from build123d import *

# Parameters (mm, degrees)
SKETCH1_R           = 42.5
SKETCH1_R_2         = 35.5
BOSS_EXTRUDE3_DEPTH = 20
BOSS_EXTRUDE4_DEPTH = 20
BOSS_EXTRUDE6_DEPTH = 20


with BuildPart() as part:
    # Sketch1 → Boss-Extrude3 (new body)
    with BuildSketch(Plane(origin=(0, 0, 0), x_dir=(1, 0, 0), z_dir=(0, 1, 0))):
        Circle(SKETCH1_R)
        Circle(SKETCH1_R_2, mode=Mode.SUBTRACT)
    extrude(amount=BOSS_EXTRUDE3_DEPTH)

    # Sketch5 → Boss-Extrude4 (add)
    with BuildSketch(Plane(origin=(0, 0, 0), x_dir=(1, 0, 0), z_dir=(0, 1, 0))):
        with BuildLine():
            Line((-30, -94.285), (30, -94.285))
            Line((30, -94.285), (30, -30.103986447))
            ThreePointArc((30, -30.103986447), (0, -42.5), (-30, -30.103986447))
            Line((-30, -30.103986447), (-30, -94.285))
        make_face()
    extrude(amount=BOSS_EXTRUDE4_DEPTH)

    # Sketch6 → Boss-Extrude6 (add)
    with BuildSketch(Plane.XY.offset(94.285)):
        with BuildLine():
            Line((70, -20), (-70, -20))
            ThreePointArc((-70, -20), (-100, 10), (-70, 40))
            Line((-70, 40), (70, 40))
            ThreePointArc((70, 40), (100, 10), (70, -20))
        make_face()
        with BuildLine():
            Line((-45, 0), (-75, 0))
            ThreePointArc((-75, 0), (-85, 10), (-75, 20))
            Line((-75, 20), (-45, 20))
            ThreePointArc((-45, 20), (-35, 10), (-45, 0))
        make_face(mode=Mode.SUBTRACT)
        with BuildLine():
            Line((45, 0), (75, 0))
            ThreePointArc((75, 0), (85, 10), (75, 20))
            Line((75, 20), (45, 20))
            ThreePointArc((45, 20), (35, 10), (45, 0))
        make_face(mode=Mode.SUBTRACT)
    extrude(amount=BOSS_EXTRUDE6_DEPTH)


solid = part.part
Can you work these out from the model? Positions are in its coordinate system, mm. A direction names the side the tool comes from. Coordinates: 2 decimals unless noted, no trailing zeros. Write each loop counter-clockwise with the first axis right and the second up, starting at its lowest first coordinate (ties: lowest second). Pieces come first, ordered by that corner, then holes. Notation, with made-up numbers: (-26, -18.75) -> (-14, -18.75) arc R23 cw to (-14, 15.25) -> close; hole circle Ø6 at (71.5, 18). An arc over 180 degrees is marked (long way). Write each question's results on one line, items separated by ' | '. Start each with the question number.
Item 1: If we section it at A-A, the plane y = 10: Write out the boundary of the cut face in (x, z) (3 decimals).
Item 2: Thinking about a two-plate mould opening in X: for faces 5 (the flat face through (-30, 10, 62)), 6 (the cylindrical face through (85, 10, 104)), 7 (the flat face through (-60, 0, 104)), 8 (the flat face through (-1, 0, 40)), which applies, released by +X, released by -X, zero draft, split by the parting line, or undercut?
Item 3: Please list where these lines run through material, in increasing order: probe 1 along X at (y, z) = (8.75, 0); probe 2 along Z at (x, y) = (0, 14) (3 decimals); probe 3 along Z at (x, y) = (-85, -2.5) (3 decimals).
Item 4: If we section it at D-D, the plane z = 98: Write out the boundary of the cut face in (x, y).
Item 5: On a 3-axis mill with a long thin cutter (end or side, diameter ignored), from which of +Z, -Z, +X, -X, +Y, -Y can I reach the whole of each face in a straight line? I mean faces 1 (the flat face through (-1, 20, 40)), 2 (the flat face through (30, 10, 63)), 3 (the cylindrical face through (35, 10, 104)), 4 (the flat face through (-60, 20, 104)). Say none if no direction works.
Item 6: If we section it at C-C, the plane x = 48: Write out the boundary of the cut face in (y, z) (3 decimals).
Item 7: I'm going to push flat-ended pins straight in: P1, Ø10, axis at y = 22.5, z = -5.5, coming from the +X side; P2, Ø6, axis at x = -46, y = 15.5, coming from the +Z side; P3, Ø6, axis at y = 14, z = 64.5, coming from the +X side; P4, Ø16, axis at y = 11, z = 77.5, coming from the -X side. Where does each tip first touch, or does it pass through?
Item 8: If we section it at B-B, the plane z = 0: Write out the boundary of the cut face in (x, y), and give its area (3 significant figures).
Answer block:
1) outline: (-100, 94.285) -> (-85, 94.285) -> (-85, 114.285) -> (-100, 114.285) -> close; (-35, 94.285) -> (-30, 94.285) -> (-30, 30.104) arc R42.5 ccw (long way) to (30, 30.104) -> (30, 94.285) -> (35, 94.285) -> (35, 114.285) -> (-35, 114.285) -> close; (85, 94.285) -> (100, 94.285) -> (100, 114.285) -> (85, 114.285) -> close; hole circle Ø71 at (0, 0)
2) face 5: released by -X | face 6: undercut | face 7: undercut | face 8: zero draft
3) probe 1: -42.5 to -35.5, 35.5 to 42.5 | probe 2: -42.5 to -35.5, 35.5 to 114.285 | probe 3: 94.285 to 114.285
4) outline: (-70, -20) -> (70, -20) arc R30 ccw to (70, 40) -> (-70, 40) arc R30 ccw to start; hole (-75, 0) -> (-45, 0) arc R10 ccw to (-45, 20) -> (-75, 20) arc R10 ccw to start; hole (45, 0) -> (75, 0) arc R10 ccw to (75, 20) -> (45, 20) arc R10 ccw to start
5) face 1: -Z, +X, -X, +Y | face 2: +X, +Y, -Y | face 3: +Z | face 4: +Z, -Z
6) outline: (-20, 94.285) -> (0, 94.285) -> (0, 114.285) -> (-20, 114.285) -> close; (20, 94.285) -> (40, 94.285) -> (40, 114.285) -> (20, 114.285) -> close
7) P1: x = 42.48 | P2: through | P3: x = 30 | P4: x = -30
8) outline: (-42.5, 0) -> (-35.5, 0) -> (-35.5, 20) -> (-42.5, 20) -> close; (35.5, 0) -> (42.5, 0) -> (42.5, 20) -> (35.5, 20) -> close | area: 280 mm²
